from build123d import *

# Parameters (mm, degrees)
CROQUIS1_R              = 8.5
CROQUIS1_R_2            = 1.5
SALIENTE_EXTRUIR1_DEPTH = 1.5
REDONDEO1_R             = 3


with BuildPart() as part:
    # Croquis1 → Saliente-Extruir1 (new body, symmetric)
    with BuildSketch(Plane(origin=(0, 0, 0), x_dir=(1, 0, 0), z_dir=(0, 1, 0))):
        Polygon((-11, 0), (11, 0), (20.5, 17.599715907), (20.5, 47.599715907), (8, 62), (-8, 62), (-20.5, 47.599715907), (-20.5, 17.599715907), align=None)
        with Locations((7.530163354, 17.782301135)):
            Circle(CROQUIS1_R, mode=Mode.SUBTRACT)
        with Locations((-5.25, 57.994261746)):
            Circle(CROQUIS1_R_2, mode=Mode.SUBTRACT)
        with Locations((-13.5, 37.599715907)):
            Circle(CROQUIS1_R_2, mode=Mode.SUBTRACT)
        with Locations((13.5, 37.599715907)):
            Circle(CROQUIS1_R_2, mode=Mode.SUBTRACT)
        with Locations((5.25, 57.994261746)):
            Circle(CROQUIS1_R_2, mode=Mode.SUBTRACT)
        with Locations((-6, 4)):
            Circle(CROQUIS1_R_2, mode=Mode.SUBTRACT)
        with Locations((6, 4)):
            Circle(CROQUIS1_R_2, mode=Mode.SUBTRACT)
        with BuildLine():
            Line((-8.730303993, 39.099715907), (8.730303993, 39.099715907))
            ThreePointArc((8.730303993, 39.099715907), (10.179901517, 41.338291312), (12.574074074, 42.513234115))
            ThreePointArc((12.574074074, 42.513234115), (0, 51.099715907), (-12.574074074, 42.513234115))
            ThreePointArc((-12.574074074, 42.513234115), (-10.179901517, 41.338291312), (-8.730303993, 39.099715907))
        make_face(mode=Mode.SUBTRACT)
        with BuildLine():
            Line((-13.5, 32.599715907), (-13.5, 17.782301135))
            ThreePointArc((-13.5, 17.782301135), (-9.234918323, 13.517219458), (-4.969836646, 17.782301135))
            ThreePointArc((-4.969836646, 17.782301135), (-0.361028795, 27.476582257), (10.06681719, 30.022210747))
            ThreePointArc((10.06681719, 30.022210747), (11.99598649, 31.106273213), (11.187975781, 33.166371344))
            ThreePointArc((11.187975781, 33.166371344), (9.667400631, 34.388612969), (8.730303993, 36.099715907))
            Line((8.730303993, 36.099715907), (-8.730303993, 36.099715907))
            ThreePointArc((-8.730303993, 36.099715907), (-10.541960108, 33.568587033), (-13.5, 32.599715907))
        make_face(mode=Mode.SUBTRACT)
    extrude(amount=SALIENTE_EXTRUIR1_DEPTH, both=True)

    # Redondeo1
    redondeo1_edges = [part.edges().sort_by_distance(p)[0] for p in [
        (-20.5, 0, -17.599715907),
        (-20.5, 0, -47.599715907),
        (-8, 0, -62),
        (8, 0, -62),
        (20.5, 0, -47.599715907),
        (20.5, 0, -17.599715907),
    ]]
    fillet(redondeo1_edges, radius=REDONDEO1_R)


solid = part.part
Design review of the part built by this model. Coordinates are the model's own, in mm. A direction names the side the tool comes from. Give positions to 0.01 mm unless a question says otherwise; leave off trailing zeros. Order: outer loops, then holes, each group sorted by start corner. A loop starts at its lowest first (then second) coordinate and runs counter-clockwise, first axis right, second up.
1. Mouldability with a two-part tool opening along X and no side actions: class faces 1 (the cylindrical face through (12.3, 0, -36.7)), 2 (the flat face through (0, -1.5, -38)), 3 (the flat face through (-20.5, 0, -33)) as +X half, -X half, draft (parallel to the pull), parting line (faces both ways), or undercut.
Solution:
face 1: undercut
face 2: draft
face 3: -X half
2. Add section C-C, the plane z = -4. State the section outline as (x, y) points.
Solution:
outline: (-13.16, -1.5) - (-7.5, -1.5) - (-7.5, 1.5) - (-13.16, 1.5) - close; (-4.5, -1.5) - (4.5, -1.5) - (4.5, 1.5) - (-4.5, 1.5) - close; (7.5, -1.5) - (13.16, -1.5) - (13.16, 1.5) - (7.5, 1.5) - close
3. Add section B-B, the plane x = 2. State the section outline as (y, z) points.
Solution:
outline: (-1.5, -62) - (1.5, -62) - (1.5, -50.95) - (-1.5, -50.95) - close; (-1.5, -39.1) - (1.5, -39.1) - (1.5, -36.1) - (-1.5, -36.1) - close; (-1.5, -28.99) - (1.5, -28.99) - (1.5, -24.24) - (-1.5, -24.24) - close; (-1.5, -11.33) - (1.5, -11.33) - (1.5, 0) - (-1.5, 0) - close
4. To check wall thickness, follow L1, parallel to X at y = -1.15, z = -3; L2, parallel to Z at x = -1, y = 0.9; L3, parallel to Z at x = -6, y = 0.55. State the ranges of each line that lie inside material, in increasing order.
Solution:
L1: x = -12.62 to -7.12, -4.88 to 4.88, 7.12 to 12.62
L2: z = -62 to -51.06, -39.1 to -36.1, -26.92 to 0
L3: z = -62 to -59.29, -56.7 to -49.69, -39.1 to -36.1, -15 to -5.5, -2.5 to 0
5. Tool access review of faces 4 (the cylindrical face through (-0.48, 0.02, -27.38)), 5 (the flat face through (20.5, 0, -32)): name each direction out of +Z, -Z, +X, -X, +Y, -Y from which nothing blocks a thin tool from reaching the whole face with its end or side.
Solution:
face 4: +Y, -Y
face 5: +Z, -Z, +X, +Y, -Y
6. Add section D-D, the plane y = 0.4. State how many separate pieces and enclosed holes the cut face has, then the cut area to 3 significant figures.
Solution:
separate pieces: 1
enclosed holes: 9
area: 1,400 mm2
7. Add section A-A, the plane x = -6. State the section outline as (y, z) points, then the cut area to 3 significant figures.
Solution:
outline: (-1.5, -62) - (1.5, -62) - (1.5, -59.29) - (-1.5, -59.29) - close; (-1.5, -56.7) - (1.5, -56.7) - (1.5, -49.69) - (-1.5, -49.69) - close; (-1.5, -39.1) - (1.5, -39.1) - (1.5, -36.1) - (-1.5, -36.1) - close; (-1.5, -15) - (1.5, -15) - (1.5, -5.5) - (-1.5, -5.5) - close; (-1.5, -2.5) - (1.5, -2.5) - (1.5, 0) - (-1.5, 0) - close
area: 74.1 mm2
8. For pin 1 Ø10 at (x, z) = (7.53, -17.78) entering from -Y; pin 2 Ø3.5 at (x, z) = (-5.25, -57.99) entering from -Y; pin 3 Ø1 at (y, z) = (-1, -48) entering from +X, all flat-tipped, find the tip position at first contact; note any pin that passes through.
Solution:
pin 1: passes through
pin 2: stops at y = -1.5
pin 3: stops at x = 20.32
